For this review, take the finished solid that the model builds, in its own axes (mm). Face numbers are marked on the shaded views. A direction names the side the tool comes from. Round coordinates to 2 decimals unless told otherwise and drop trailing zeros. Write each loop counter-clockwise with the first axis right and the second up, starting at its lowest first coordinate (ties: lowest second). Pieces come first, ordered by that corner, then holes. Notation, with made-up numbers: M -2,-39.75 L 46,-39.75 A10 cw 46,-30.75 Z; hole C 39,14 d3. An arc over 180 degrees is marked long. One line per question, with ' | ' between items.
```python
from build123d import *

# Parameters (mm, degrees)
SKETCH1_R           = 3.75
BOSS_EXTRUDE1_DEPTH = 5
CUT_EXTRUDE2_DEPTH  = 2
SKETCH5_R           = 0.8
SKETCH5_W           = 12.2
SKETCH5_H           = 23.2
BOSS_EXTRUDE2_DEPTH = 4
FILLET1_R           = 3


with BuildPart() as part:
    # Sketch1 → Boss-Extrude1 (new body)
    with BuildSketch(Plane.XY):
        with BuildLine():
            Line((10, -17.5), (-5, -17.5))
            ThreePointArc((-5, -17.5), (-8.535533906, -16.035533906), (-10, -12.5))
            Line((-10, -12.5), (-10, 12.5))
            ThreePointArc((-10, 12.5), (-8.535533906, 16.035533906), (-5, 17.5))
            Line((-5, 17.5), (10, 17.5))
            Line((10, 17.5), (10, -17.5))
        make_face()
        Circle(SKETCH1_R, mode=Mode.SUBTRACT)
    extrude(amount=-BOSS_EXTRUDE1_DEPTH)

    # Sketch3 → Cut-Extrude2 (cut)
    with BuildSketch(Plane.XY):
        with BuildLine():
            Line((-1.984313483, 14.25), (-3.720587781, 0.46875))
            ThreePointArc((-3.720587781, 0.46875), (-3.75, 0), (-3.720587781, -0.46875))
            Line((-3.720587781, -0.46875), (-1.984313483, -14.25))
            ThreePointArc((-1.984313483, -14.25), (0, -16), (1.984313483, -14.25))
            Line((1.984313483, -14.25), (3.720587781, -0.46875))
            ThreePointArc((3.720587781, -0.46875), (3.75, 0), (3.720587781, 0.46875))
            Line((3.720587781, 0.46875), (1.984313483, 14.25))
            ThreePointArc((1.984313483, 14.25), (0, 16), (-1.984313483, 14.25))
        make_face()
    extrude(amount=-CUT_EXTRUDE2_DEPTH, mode=Mode.SUBTRACT)

    # Sketch5 → Boss-Extrude2 (add)
    with BuildSketch(Plane(origin=(10, 0, 0), x_dir=(0, 0, -1), z_dir=(1, 0, 0))):
        with BuildLine():
            Line((5, 17.5), (-10.2, 17.5))
            ThreePointArc((-10.2, 17.5), (-13.735533906, 16.035533906), (-15.2, 12.5))
            Line((-15.2, 12.5), (-15.2, -12.5))
            ThreePointArc((-15.2, -12.5), (-13.735533906, -16.035533906), (-10.2, -17.5))
            Line((-10.2, -17.5), (5, -17.5))
            Line((5, -17.5), (5, 17.5))
        make_face()
        with Locations((-7.1, 13.85)):
            Circle(SKETCH5_R, mode=Mode.SUBTRACT)
        with Locations((-7.1, -13.85)):
            Circle(SKETCH5_R, mode=Mode.SUBTRACT)
        with Locations((-7.1, 0)):
            Rectangle(SKETCH5_W, SKETCH5_H, mode=Mode.SUBTRACT)
    extrude(amount=-BOSS_EXTRUDE2_DEPTH)

    # Fillet1
    fillet1_edges = [part.edges().sort_by_distance(p)[0] for p in [
        (10, 0, -5),
    ]]
    fillet(fillet1_edges, radius=FILLET1_R)


solid = part.part
```
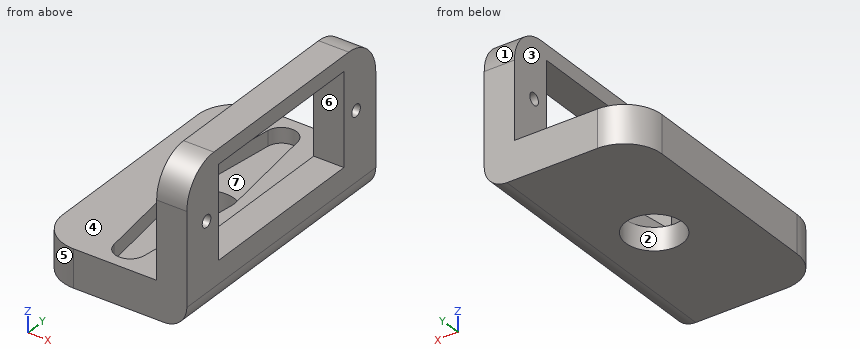
Item 1: To check wall thickness, follow line 1 along Y through (x, z) = (7.6, 7.1); line 2 along Y through (x, z) = (0, -3.6); line 3 along Z through (x, y) = (6.75, -5). State the ranges of each line that lie inside material, in increasing order. Write a range as from..to.
Results:
line 1: -17.5..-14.65, -13.05..-11.6, 11.6..13.05, 14.65..17.5 | line 2: -17.5..-3.75, 3.75..17.5 | line 3: -5..1, 13.2..15.2
Item 2: Machinability: for the marked faces 4, 5, 6 and 7, which of the approach directions +Z, -Z, +X, -X, +Y, -Y give a long, thin tool a straight path to every point of the face, cutting with its end or side? Answer none if there is none.
Results:
face 4: +Z, -X, +Y, -Y | face 5: +Z, -Z, -X, -Y | face 6: +X, -X | face 7: +Z
Item 3: Take a section at B-B (y = 13.85). Write out the cut boundary in (x, z).
Results:
outline: M -9.81,-5 L 7,-5 A3 ccw 10,-2 L 10,6.3 L 6,6.3 L 6,0 L 2.03,0 L 2.03,-2 L -2.03,-2 L -2.03,0 L -9.81,0 Z; M 6,7.9 L 10,7.9 L 10,15.01 L 6,15.01 Z
Item 4: Mouldability with a two-part tool opening along X and no side actions: class the marked faces 1, 2 and 3 as +X half, -X half, draft (parallel to the pull), parting line (faces both ways), or undercut.
Results:
face 1: draft | face 2: undercut | face 3: -X half
Item 5: Take a section at D-D (z = 4). Write out the cut boundary in (x, y), then the cut area to 3 significant figures.
Results:
outline: M 6,-17.5 L 10,-17.5 L 10,-11.6 L 6,-11.6 Z; M 6,11.6 L 10,11.6 L 10,17.5 L 6,17.5 Z | area: 47.2 mm2
Item 6: Take a section at C-C (x = 0). Write out the cut boundary in (y, z).
Results:
outline: M -17.5,-5 L -3.75,-5 L -3.75,-2 L -16,-2 L -16,0 L -17.5,0 Z; M 3.75,-5 L 17.5,-5 L 17.5,0 L 16,0 L 16,-2 L 3.75,-2 Z
Item 7: Take a section at A-A (z = 7.1). Write out the cut boundary in (x, y).
Results:
outline: M 6,-17.5 L 10,-17.5 L 10,-14.65 L 6,-14.65 Z; M 6,-13.05 L 10,-13.05 L 10,-11.6 L 6,-11.6 Z; M 6,11.6 L 10,11.6 L 10,13.05 L 6,13.05 Z; M 6,14.65 L 10,14.65 L 10,17.5 L 6,17.5 Z
Item 8: Insertion check: pin 1 Ø2 at (y, z) = (-13.85, 7.1) entering from -X; pin 2 Ø4 at (x, y) = (-2.5, -1.5) entering from +Z; pin 3 Ø1.4 at (y, z) = (13.85, 7.1) entering from -X; pin 4 Ø12 at (x, z) = (3.5, 10) entering from +Y. Each pin has a flat end and moves straight along its axis. Give the tip position at first contact, or say it passes through.
Results:
pin 1: x = 6 | pin 2: z = 0 | pin 3: through | pin 4: y = 17.5
